Source: CAD feature listing. Evaluate the final solid. Frame: model axes, mm. Give positions to 0.01 mm unless a question says otherwise; leave off trailing zeros. Loops run counter-clockwise (first coordinate to the right, second up) from the corner with the lowest first, then second, coordinate; pieces in that order, holes last. Notation, with made-up numbers: (-9, -23) -> (10, -23) arc R29 cw to (10, 6) -> close; hole circle Ø9 at (78, 19.25). An arc over 180 degrees is marked (long way). Answer as a JSON object with one key per item and string values. Group by question number.
from build123d import *

# Parameters (mm, degrees)
BOSS_EXTRUDE2_DEPTH       = 3
M4X0_7_TAPPED_HOLE2_D     = 3.3
M4X0_7_TAPPED_HOLE2_DEPTH = 10.1
M4X0_7_TAPPED_HOLE2_TIP   = 0.991420021


with BuildPart() as part:
    # Sketch1 → Boss-Extrude2 (new body)
    with BuildSketch(Plane(origin=(0, 0, 0), x_dir=(1, 0, 0), z_dir=(0, 1, 0))):
        with BuildLine():
            Line((-28, 6), (0, 6))
            ThreePointArc((0, 6), (6, 0), (0, -6))
            Line((0, -6), (-28, -6))
            ThreePointArc((-28, -6), (-34, 0), (-28, 6))
        make_face()
    extrude(amount=BOSS_EXTRUDE2_DEPTH)

    # M4x0.7 Tapped Hole2
    with Locations(Plane(origin=(0, 3, 0), x_dir=(1, 0, 0), z_dir=(0, 1, 0))):
        with Locations((0, 0), (-14, 0), (-28, 0)):
            Hole(M4X0_7_TAPPED_HOLE2_D / 2, depth=M4X0_7_TAPPED_HOLE2_DEPTH)
            with Locations((0, 0, -(M4X0_7_TAPPED_HOLE2_DEPTH + M4X0_7_TAPPED_HOLE2_TIP / 2))):  # 118° drill point
                Cone(0, M4X0_7_TAPPED_HOLE2_D / 2, M4X0_7_TAPPED_HOLE2_TIP, mode=Mode.SUBTRACT)


solid = part.part
(1) Section query A-A on z = 0. Return the cut outline in (x, y), plus the area to 3 significant figures.
(2) Section query D-D on x = -29. Return the cut outline in (y, z).
(3) Material intervals for line 1 (Z direction, x = -14, y = 1.9); line 2 (X direction, y = 1.3, z = 1); line 3 (X direction, y = 0.7, z = -1.25), sorted ascending. Write a range as from..to.
(4) Section query C-C on y = 1.35. Return the cut outline in (x, z).
(5) Section query B-B on x = -14. Return the cut outline in (y, z), plus the area to 3 significant figures.
(6) Mould query, pull axis Z, two halves, no side actions, for faces 1 (the face through (-14, 1, 6)), 2 (the face through (-26.35, 1.48, -0.07)), 3 (the face through (-14, 1, -6)). Classes: pulls with the +Z half, pulls with the -Z half, needs draft (parallel to the pull), parting line crosses it, or undercut.
(7) First-contact query: pin 1 (1.5 mm diameter, centred on x = 1.5, y = 1, fed in from +Z); pin 2 (6 mm diameter, centred on x = -18.5, z = -1.5, fed in from -Y). Flat tips, straight axial feed; report the tip coordinate or a pass-through.
Result:
{
 "1": {"outline": "(-34, 0) -> (-29.65, 0) -> (-29.65, 3) -> (-34, 3) -> close; (-26.35, 0) -> (-15.65, 0) -> (-15.65, 3) -> (-26.35, 3) -> close; (-12.35, 0) -> (-1.65, 0) -> (-1.65, 3) -> (-12.35, 3) -> close; (1.65, 0) -> (6, 0) -> (6, 3) -> (1.65, 3) -> close", "area": "90.3 mm²"},
 "2": {"outline": "(0, -5.92) -> (3, -5.92) -> (3, -1.31) -> (0, -1.31) -> close; (0, 1.31) -> (3, 1.31) -> (3, 5.92) -> (0, 5.92) -> close"},
 "3": {"line 1": "-6..-1.65, 1.65..6", "line 2": "-33.92..-29.31, -26.69..-15.31, -12.69..-1.31, 1.31..5.92", "line 3": "-33.87..-29.08, -26.92..-15.08, -12.92..-1.08, 1.08..5.87"},
 "4": {"outline": "(-28, -6) -> (0, -6) arc R6 ccw to (0, 6) -> (-28, 6) arc R6 ccw to start; hole circle Ø3.3 at (-28, 0); hole circle Ø3.3 at (-14, 0); hole circle Ø3.3 at (0, 0)"},
 "5": {"outline": "(0, -6) -> (3, -6) -> (3, -1.65) -> (0, -1.65) -> close; (0, 1.65) -> (3, 1.65) -> (3, 6) -> (0, 6) -> close", "area": "26.1 mm²"},
 "6": {"face 1": "pulls with the +Z half", "face 2": "undercut", "face 3": "pulls with the -Z half"},
 "7": {"pin 1": "z = 5.95", "pin 2": "y = 0"}
}
